Source: three-view drawing plus pictorial views. Frame: mm from the lowest corner of the part. Give positions to 0.01 mm unless a question says otherwise; leave off trailing zeros. Loops run counter-clockwise (first coordinate to the right, second up) from the corner with the lowest first, then second, coordinate; pieces in that order, holes last. Notation, with made-up numbers: (37, 6.25) -> (77, 6.25) arc R12 ccw to (77, 23.25) -> close; hole circle Ø1 at (8.25, 61.5). An arc over 180 degrees is marked (long way). Answer as a JSON object with one key per item and string values. Group by question number.
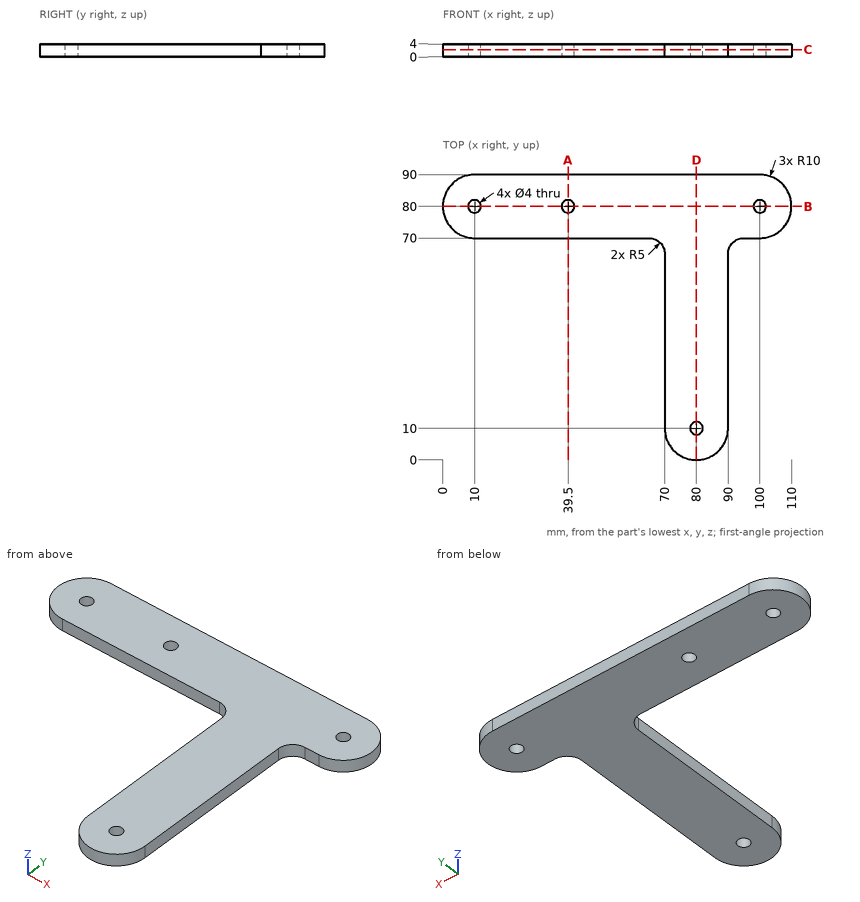
(1) First-contact query: pin 1 (2 mm diameter, centred on y = 50.5, z = 2, fed in from -X); pin 2 (1.5 mm diameter, centred on y = 60, z = 0.5, fed in from +X); pin 3 (5 mm diameter, centred on x = 10, y = 80, fed in from -Z); pin 4 (3.5 mm diameter, centred on x = 80, y = 10, fed in from -Z). Flat tips, straight axial feed; report the tip coordinate or a pass-through.
(2) Section query D-D on x = 80. Return the cut outline in (y, z).
(3) Section query B-B on y = 80. Return the cut outline in (x, z).
(4) Material intervals for line 1 (Y direction, x = 80, z = 2.15); line 2 (Y direction, x = 10, z = 1.9); line 3 (X direction, y = 31, z = 1.4), sorted ascending. Write a range as from..to.
(5) Section query C-C on z = 2.25. Return the cut outline in (x, y), plus the area to 3 significant figures.
(6) Section query A-A on x = 39.5. Return the cut outline in (y, z), plus the area to 3 significant figures.
Result:
{
 "1": {"pin 1": "x = 70", "pin 2": "x = 90", "pin 3": "z = 0", "pin 4": "through"},
 "2": {"outline": "(0, 0) -> (8, 0) -> (8, 4) -> (0, 4) -> close; (12, 0) -> (90, 0) -> (90, 4) -> (12, 4) -> close"},
 "3": {"outline": "(0, 0) -> (8, 0) -> (8, 4) -> (0, 4) -> close; (12, 0) -> (37.5, 0) -> (37.5, 4) -> (12, 4) -> close; (41.5, 0) -> (98, 0) -> (98, 4) -> (41.5, 4) -> close; (102, 0) -> (110, 0) -> (110, 4) -> (102, 4) -> close"},
 "4": {"line 1": "0..8, 12..90", "line 2": "70..78, 82..90", "line 3": "70..90"},
 "5": {"outline": "(10, 70) -> (65, 70) arc R5 cw to (70, 65) -> (70, 10) arc R10 ccw to (90, 10) -> (90, 65) arc R5 cw to (95, 70) -> (100, 70) arc R10 ccw to (100, 90) -> (10, 90) arc R10 ccw to start; hole circle Ø4 at (10, 80); hole circle Ø4 at (39.5, 80); hole circle Ø4 at (80, 10); hole circle Ø4 at (100, 80)", "area": "3,430 mm²"},
 "6": {"outline": "(70, 0) -> (78, 0) -> (78, 4) -> (70, 4) -> close; (82, 0) -> (90, 0) -> (90, 4) -> (82, 4) -> close", "area": "64.0 mm²"}
}
